Could you check a few things on this model? Use its own coordinates, in mm. A direction names the side the tool comes from. Round coordinates to 2 decimals unless told otherwise and drop trailing zeros. Loops run counter-clockwise (first coordinate to the right, second up) from the corner with the lowest first, then second, coordinate; pieces in that order, holes last. Notation, with made-up numbers: (88.25, 28) -> (109.25, 28) arc R9 cw to (109.25, 32) -> close; hole circle Ø10 at (61, 65). An arc over 180 degrees is marked (long way). One line per item, written item: value.
```python
from build123d import *

# Parameters (mm, degrees)
F0_W           = 25.4
F0_H           = 10.16
F1_DEPTH       = 12.7
F3_DEPTH       = 19.812
F5_D           = 4.4958
F5_CBORE_D     = 6.6294
F5_CBORE_DEPTH = 2.54
F7_D           = 3.571875
F7_CBORE_D     = 6.746875
F7_CBORE_DEPTH = 6.1722
F8_D           = 3.4544
F8_DEPTH       = 6.35
F8_TIP         = 1.0378064612
F9_D           = 3.048


with BuildPart() as f1:
    # F0 (on Top) → F1 (new body)
    with BuildSketch(Plane.XY):
        with Locations((12.7, 5.08)):
            Rectangle(F0_W, F0_H)
    extrude(amount=F1_DEPTH)

    # F2 (on face) → F3 (join)
    with BuildSketch(Plane(origin=(0, 0, 0), x_dir=(1, 0, 0), z_dir=(0, 0, -1))):
        Polygon((8.8914105889, 0), (6.985, -3.302), (18.415, -3.302), (16.5085894111, 0), align=None)
    extrude(amount=F3_DEPTH)

    # F5 (through all)
    with Locations(Plane.XZ):
        with Locations((5.08, 7.62), (20.32, 7.62)):
            CounterBoreHole(F5_D / 2, F5_CBORE_D / 2, F5_CBORE_DEPTH)

    # F7 (through all)
    with Locations(Plane.XY.offset(12.7)):
        with Locations((12.7, 6.35)):
            CounterBoreHole(F7_D / 2, F7_CBORE_D / 2, F7_CBORE_DEPTH)

    # F8
    with Locations(Plane.XZ):
        with Locations((12.7, 9.652)):
            Hole(F8_D / 2, depth=F8_DEPTH)
            with Locations((0, 0, -(F8_DEPTH + F8_TIP / 2))):  # 118° drill point
                Cone(0, F8_D / 2, F8_TIP, mode=Mode.SUBTRACT)

    # F9 (through all)
    with Locations(Plane.XZ):
        with Locations((12.7, 9.652)):
            Hole(F9_D / 2)


solid = f1.part
```
Item 1: I need wall thicknesses on line 1 (Z direction, x = 5.08, y = 1.2); line 2 (Z direction, x = 20.32, y = 6.75); line 3 (Y direction, x = 12.25, z = -13). Which ranges of each line are inside material? Lowest first, please. Write a range as from..to.
Output:
line 1: z = 0..4.31, 10.93..12.7
line 2: z = 0..5.37, 9.87..12.7
line 3: y = 0..3.3
Item 2: Will these pins go through, and if not, where does the flat tip stop? pin 1 Ø6 at (x, y) = (8, 4.5) entering from -Z; pin 2 Ø1 at (x, y) = (3.5, 7.5) entering from -Z; pin 3 Ø5 at (x, z) = (20.32, 7.62) entering from -Y; pin 4 Ø3 at (x, y) = (12.7, 6.35) entering from -Z.
Output:
pin 1: stops at z = -19.81
pin 2: stops at z = 0
pin 3: stops at y = 2.54
pin 4: passes through
Item 3: If we section it at A-A on y = 6.35: List the corners of the cut face in (x, z) for me, plus the area to 3 significant figures.
Output:
outline: (0, 0) -> (10.91, 0) -> (10.91, 6.53) -> (9.33, 6.53) -> (9.33, 12.7) -> (0, 12.7) -> close; (14.49, 0) -> (25.4, 0) -> (25.4, 12.7) -> (16.07, 12.7) -> (16.07, 6.53) -> (14.49, 6.53) -> close; hole circle Ø4.5 at (5.08, 7.62); hole circle Ø4.5 at (20.32, 7.62)
area: 226 mm²
Item 4: If we section it at C-C on x = 20.32: List the corners of the cut face in (y, z) for me, plus the area to 3 significant figures.
Output:
outline: (0, 0) -> (10.16, 0) -> (10.16, 5.37) -> (2.54, 5.37) -> (2.54, 4.31) -> (0, 4.31) -> close; (0, 10.93) -> (2.54, 10.93) -> (2.54, 9.87) -> (10.16, 9.87) -> (10.16, 12.7) -> (0, 12.7) -> close
area: 77.9 mm²
Item 5: If we section it at B-B on x = 12.7: List the corners of the cut face in (y, z) for me, plus the area to 3 significant figures.
Output:
outline: (0, -19.81) -> (3.3, -19.81) -> (3.3, 0) -> (4.56, 0) -> (4.56, 6.53) -> (2.98, 6.53) -> (2.98, 7.92) -> (0, 7.92) -> close; (0, 11.38) -> (2.98, 11.38) -> (2.98, 12.7) -> (0, 12.7) -> close; (8.14, 0) -> (10.16, 0) -> (10.16, 8.13) -> (9.72, 8.13) -> (9.72, 6.53) -> (8.14, 6.53) -> close; (9.72, 11.18) -> (10.16, 11.18) -> (10.16, 12.7) -> (9.72, 12.7) -> close
area: 118 mm²
Item 6: If we section it at D-D on z = 3: List the corners of the cut face in (x, y) for me, plus the area to 3 significant figures.
Output:
outline: (0, 0) -> (25.4, 0) -> (25.4, 10.16) -> (0, 10.16) -> close; hole circle Ø3.57 at (12.7, 6.35)
area: 248 mm²
Item 7: For faces 4 (the face through (23.4, 1.3, 6.4)), 5 (the face through (14.514, 9.194, 9.657)), 6 (the face through (17.475, 1.674, -9.767)), 7 (the face through (0, 5, 6)), which set-ups out of +Z, -Z, +X, -X, +Y, -Y let a thin tool reach every point of the face, with its end or its side?
Output:
face 4: -Y
face 5: +Z
face 6: -Z, +X, -Y
face 7: +Z, -Z, -X, +Y, -Y
Item 8: If we mould it in two halves opening along Y, with no side actions, what happens to faces 1 (the face through (13, 3.302, -10)), 2 (the face through (14.2, 4.9, 6.528)), 3 (the face through (2.45, 1.25, 5.6))? For each: released by +Y, released by -Y, zero draft, split by the parting line, or undercut.
Output:
face 1: released by +Y
face 2: undercut
face 3: zero draft
